Autodesk Inventor part; units mm, degrees
ref_plane "YZ Plane" through (0, 0, 0) normal (1, 0, 0) x (0, 1, 0)
ref_plane "XZ Plane" through (0, 0, 0) normal (0, 1, 0) x (-1, 0, 0)
ref_plane "XY Plane" through (0, 0, 0) normal (0, 0, 1) x (1, 0, 0)
sketch "Sketch1" plane through (0, 0, 0) normal (0, 0, 1) x (1, 0, 0)
  line L0 (0, 0) -> (300, 0)
  line L1 (300, 0) -> (300, 62)
  line L2 (300, 62) -> (0, 62)
  line L3 (0, 62) -> (0, 0)
  circle A0 centre (144.5, 55.5) radius 1.55
  circle A1 centre (144.5, 24.5) radius 1.55
  circle A2 centre (175.5, 55.5) radius 1.55
  circle A3 centre (175.5, 24.5) radius 1.55
  circle A4 centre (160, 40) radius 11.5
  line L4 (5, 19) -> (140, 19)
  line L5 (140, 19) -> (140, 15)
  line L6 (140, 15) -> (5, 15)
  line L7 (5, 15) -> (5, 19)
  line L8 (0, 62) -> (39.6145, 62)
  line L9 (8.1, 24.8) -> (5, 24.8)
  line L10 (5, 24.8) -> (5, 55.2)
  line L11 (5, 55.2) -> (8.1, 55.2)
  line L12 (8.1, 55.2) -> (8.1, 24.8)
  line L13 (8.1, 24.8) -> (5, 55.2) construction
  line L14 (5, 24.8) -> (8.1, 55.2) construction
  line L15 (0, 62) -> (50, 62)
  line L16 (0, 0) -> (0, -10)
  line L17 (0, -10) -> (300, -10)
  line L18 (300, -10) -> (300, 0)
  point P0 (6.55, 40)
  point P1 (5, 40)
  point P2 (8.1, 40)
  point P3 (5, 17)
  point P4 (140, 17)
  dimension "d1" = 3.1
  dimension "d2" = 3.1
  dimension "d3" = 3.1
  dimension "d4" = 3.1
  dimension "d5" = 31
  dimension "d7" = 23
  dimension "d8" = 15.5
  dimension "d9" = 15.5
  dimension "d10" = 62
  dimension "d11" = 31
  dimension "d13" = 40
  dimension "d54" = 300
  dimension "d55" = 3.1
  dimension "d56" = 5
  dimension "d57" = 15.2
  dimension "d59" = 135
  dimension "d93" = 15
  dimension "d106" = 20
  dimension "d107" = 5
  dimension "d201" = 4
  dimension "d202" = 10
extrude "Extrusion1" add sketch "Sketch1" along normal blind 3
sketch "Sketch4" plane through (0, 0, 3) normal (0, 0, 1) x (1, 0, 0)
  line L0 (300, 62) -> (0, 62)
  line L1 (244, 62) -> (248, 72)
  line L2 (248, 72) -> (254, 72)
  line L3 (254, 72) -> (250, 62)
  line L4 (0, -10) -> (300, -10)
  point P0 (0, 0)
  dimension "d108" = 10
  dimension "d109" = 4
  dimension "d110" = 50
  dimension "d111" = 6
extrude "Extrusion4" add sketch "Sketch4" against normal blind 3
sketch "Sketch7" plane through (0, 0, 3) normal (0, 0, 1) x (1, 0, 0)
  line L0 (134.4, 59.6) -> (137.6, 59.6)
  line L1 (137.6, 59.6) -> (137.6, 44.4)
  line L2 (137.6, 44.4) -> (134.4, 44.4)
  line L3 (134.4, 44.4) -> (134.4, 59.6)
  line L4 (134.4, 59.6) -> (137.6, 44.4) construction
  line L5 (137.6, 59.6) -> (134.4, 44.4) construction
  line L6 (134.4, 32.1) -> (137.6, 32.1)
  line L7 (137.6, 32.1) -> (137.6, 21.9)
  line L8 (137.6, 21.9) -> (134.4, 21.9)
  line L9 (134.4, 21.9) -> (134.4, 32.1)
  line L10 (134.4, 32.1) -> (137.6, 21.9) construction
  line L11 (137.6, 32.1) -> (134.4, 21.9) construction
  line L12 (244, 62) -> (0, 62)
  circle A0 centre (144.5, 55.5) radius 1.55
  line L13 (124.4, 59.6) -> (127.6, 59.6)
  line L14 (127.6, 59.6) -> (127.6, 44.4)
  line L15 (127.6, 44.4) -> (124.4, 44.4)
  line L16 (124.4, 44.4) -> (124.4, 59.6)
  line L17 (124.4, 59.6) -> (127.6, 44.4) construction
  line L18 (127.6, 59.6) -> (124.4, 44.4) construction
  line L19 (124.4, 32.1) -> (127.6, 32.1)
  line L20 (127.6, 32.1) -> (127.6, 21.9)
  line L21 (127.6, 21.9) -> (124.4, 21.9)
  line L22 (124.4, 21.9) -> (124.4, 32.1)
  line L23 (124.4, 32.1) -> (127.6, 21.9) construction
  line L24 (127.6, 32.1) -> (124.4, 21.9) construction
  line L25 (114.4, 59.6) -> (117.6, 59.6)
  line L26 (117.6, 59.6) -> (117.6, 44.4)
  line L27 (117.6, 44.4) -> (114.4, 44.4)
  line L28 (114.4, 44.4) -> (114.4, 59.6)
  line L29 (114.4, 59.6) -> (117.6, 44.4) construction
  line L30 (117.6, 59.6) -> (114.4, 44.4) construction
  line L31 (114.4, 32.1) -> (117.6, 32.1)
  line L32 (117.6, 32.1) -> (117.6, 21.9)
  line L33 (117.6, 21.9) -> (114.4, 21.9)
  line L34 (114.4, 21.9) -> (114.4, 32.1)
  line L35 (114.4, 32.1) -> (117.6, 21.9) construction
  line L36 (117.6, 32.1) -> (114.4, 21.9) construction
  line L37 (104.4, 59.6) -> (107.6, 59.6)
  line L38 (107.6, 59.6) -> (107.6, 44.4)
  line L39 (107.6, 44.4) -> (104.4, 44.4)
  line L40 (104.4, 44.4) -> (104.4, 59.6)
  line L41 (104.4, 59.6) -> (107.6, 44.4) construction
  line L42 (107.6, 59.6) -> (104.4, 44.4) construction
  line L43 (104.4, 32.1) -> (107.6, 32.1)
  line L44 (107.6, 32.1) -> (107.6, 21.9)
  line L45 (107.6, 21.9) -> (104.4, 21.9)
  line L46 (104.4, 21.9) -> (104.4, 32.1)
  line L47 (104.4, 32.1) -> (107.6, 21.9) construction
  line L48 (107.6, 32.1) -> (104.4, 21.9) construction
  line L49 (94.4, 59.6) -> (97.6, 59.6)
  line L50 (97.6, 59.6) -> (97.6, 44.4)
  line L51 (97.6, 44.4) -> (94.4, 44.4)
  line L52 (94.4, 44.4) -> (94.4, 59.6)
  line L53 (94.4, 59.6) -> (97.6, 44.4) construction
  line L54 (97.6, 59.6) -> (94.4, 44.4) construction
  line L55 (94.4, 32.1) -> (97.6, 32.1)
  line L56 (97.6, 32.1) -> (97.6, 21.9)
  line L57 (97.6, 21.9) -> (94.4, 21.9)
  line L58 (94.4, 21.9) -> (94.4, 32.1)
  line L59 (94.4, 32.1) -> (97.6, 21.9) construction
  line L60 (97.6, 32.1) -> (94.4, 21.9) construction
  line L61 (134.4, 10.1) -> (137.6, 10.1)
  line L62 (137.6, 10.1) -> (137.6, -0.1)
  line L63 (137.6, -0.1) -> (134.4, -0.1)
  line L64 (134.4, -0.1) -> (134.4, 10.1)
  line L65 (134.4, 10.1) -> (137.6, -0.1) construction
  line L66 (137.6, 10.1) -> (134.4, -0.1) construction
  line L67 (127.6, 10.1) -> (127.6, -0.1)
  line L68 (127.6, -0.1) -> (124.4, -0.1)
  line L69 (124.4, 10.1) -> (127.6, 10.1)
  line L70 (124.4, -0.1) -> (124.4, 10.1)
  line L71 (124.4, 10.1) -> (127.6, -0.1) construction
  line L72 (127.6, 10.1) -> (124.4, -0.1) construction
  line L73 (117.6, 10.1) -> (117.6, -0.1)
  line L74 (117.6, -0.1) -> (114.4, -0.1)
  line L75 (114.4, 10.1) -> (117.6, 10.1)
  line L76 (114.4, -0.1) -> (114.4, 10.1)
  line L77 (114.4, 10.1) -> (117.6, -0.1) construction
  line L78 (117.6, 10.1) -> (114.4, -0.1) construction
  line L79 (107.6, 10.1) -> (107.6, -0.1)
  line L80 (107.6, -0.1) -> (104.4, -0.1)
  line L81 (104.4, 10.1) -> (107.6, 10.1)
  line L82 (104.4, -0.1) -> (104.4, 10.1)
  line L83 (104.4, 10.1) -> (107.6, -0.1) construction
  line L84 (107.6, 10.1) -> (104.4, -0.1) construction
  line L85 (97.6, 10.1) -> (97.6, -0.1)
  line L86 (97.6, -0.1) -> (94.4, -0.1)
  line L87 (94.4, 10.1) -> (97.6, 10.1)
  line L88 (94.4, -0.1) -> (94.4, 10.1)
  line L89 (94.4, 10.1) -> (97.6, -0.1) construction
  line L90 (97.6, 10.1) -> (94.4, -0.1) construction
  line L91 (0, -10) -> (300, -10)
  line L92 (300, -10) -> (300, 62)
  point P0 (0, 0)
  point P1 (136, 52)
  point P2 (136, 27)
  point P3 (126, 52)
  point P4 (126, 27)
  point P5 (116, 52)
  point P6 (116, 27)
  point P7 (106, 52)
  point P8 (106, 27)
  point P9 (96, 52)
  point P10 (96, 27)
  point P11 (134.4, 52)
  point P12 (114.4, 52)
  point P13 (136, 5)
  point P14 (126, 5)
  point P15 (116, 5)
  point P16 (106, 5)
  point P17 (96, 5)
  point P18 (134.4, 5)
  point P19 (114.4, 5)
  point P20 (150, -10)
  dimension "d147" = 3.2
  dimension "d148" = 15.2
  dimension "d149" = 10.2
  dimension "d150" = 25
  dimension "d151" = 10
  dimension "d153" = 3.2
  dimension "d154" = 15.2
  dimension "d155" = 10.2
  dimension "d156" = 25
  dimension "d157" = 3.2
  dimension "d158" = 15.2
  dimension "d159" = 10.2
  dimension "d160" = 25
  dimension "d161" = 3.2
  dimension "d162" = 15.2
  dimension "d163" = 10.2
  dimension "d164" = 25
  dimension "d165" = 3.2
  dimension "d166" = 15.2
  dimension "d167" = 10.2
  dimension "d168" = 25
  dimension "d169" = 10
  dimension "d170" = 10
  dimension "d171" = 10
  dimension "d172" = 10
  dimension "d181" = 3.2
  dimension "d183" = 3.2
  dimension "d185" = 3.2
  dimension "d187" = 3.2
  dimension "d189" = 3.2
  dimension "d191" = 10
  dimension "d192" = 10
  dimension "d193" = 10
  dimension "d194" = 10
  dimension "d234" = 15
  dimension "d235" = 10.2
  dimension "d245" = 164
extrude "Extrusion6" cut sketch "Sketch7" against normal blind 3 contours L0 L1 L2 L3 | L6 L7 L8 L9 | L13 L14 L15 L16 | L19 L20 L21 L22 | L25 L26 L27 L28 | L31 L32 L33 L34 | L37 L38 L39 L40 | L43 L44 L45 L46 | L49 L50 L51 L52 | L55 L56 L57 L58 | L61 L62 L63 L64 | L67 L68 L70 L69 | L73 L74 L76 L75 | L79 L80 L82 L81 | L85 L86 L88 L87
sketch "Sketch8" plane through (0, 0, 3) normal (0, 0, 1) x (1, 0, 0)
  line L0 (0, -10) -> (300, -10)
  line L1 (279.8, 18) -> (290, 18)
  line L2 (290, 18) -> (290, 14.8)
  line L3 (290, 14.8) -> (279.8, 14.8)
  line L4 (279.8, 14.8) -> (279.8, 18)
  line L5 (300, -10) -> (300, 62)
  line L6 (4, 11.2) -> (7.2, 11.2)
  line L7 (7.2, 11.2) -> (7.2, -4)
  line L8 (7.2, -4) -> (4, -4)
  line L9 (4, -4) -> (4, 11.2)
  line L10 (4, 11.2) -> (7.2, -4) construction
  line L11 (7.2, 11.2) -> (4, -4) construction
  line L12 (282.4, 10.1) -> (285.6, 10.1)
  line L13 (285.6, 10.1) -> (285.6, -0.1)
  line L14 (285.6, -0.1) -> (282.4, -0.1)
  line L15 (282.4, -0.1) -> (282.4, 10.1)
  line L16 (282.4, 10.1) -> (285.6, -0.1) construction
  line L17 (285.6, 10.1) -> (282.4, -0.1) construction
  line L18 (274.4, 10.1) -> (277.6, 10.1)
  line L19 (277.6, 10.1) -> (277.6, -0.1)
  line L20 (277.6, -0.1) -> (274.4, -0.1)
  line L21 (274.4, -0.1) -> (274.4, 10.1)
  line L22 (274.4, 10.1) -> (277.6, -0.1) construction
  line L23 (277.6, 10.1) -> (274.4, -0.1) construction
  line L24 (97.6, -2.45) -> (282.4, -2.45)
  line L25 (282.4, -2.45) -> (282.4, -5.55)
  line L26 (282.4, -5.55) -> (97.6, -5.55)
  line L27 (97.6, -5.55) -> (97.6, -2.45)
  line L28 (97.6, -2.45) -> (282.4, -5.55) construction
  line L29 (282.4, -2.45) -> (97.6, -5.55) construction
  line L30 (137.6, 10.1) -> (137.6, -0.1)
  line L31 (290.4, 12.2) -> (293.6, 12.2)
  line L32 (293.6, 12.2) -> (293.6, -3)
  line L33 (293.6, -3) -> (290.4, -3)
  line L34 (290.4, -3) -> (290.4, 12.2)
  line L35 (290.4, 12.2) -> (293.6, -3) construction
  line L36 (293.6, 12.2) -> (290.4, -3) construction
  point P0 (0, 0)
  point P1 (5.6, 3.6)
  point P2 (4, 3.6)
  point P3 (284, 5)
  point P4 (282.4, 5)
  point P5 (276, 5)
  point P6 (274.4, 5)
  point P7 (190, -4)
  point P8 (137.6, 5)
  point P9 (97.6, -0.1)
  point P10 (292, 4.6)
  dimension "d219" = 28
  dimension "d220" = 3.2
  dimension "d221" = 10.2
  dimension "d222" = 10
  dimension "d223" = 3.2
  dimension "d224" = 15.2
  dimension "d225" = 4
  dimension "d226" = 6
  dimension "d227" = 3.2
  dimension "d229" = 3.2
  dimension "d232" = 8
  dimension "d233" = 15
  dimension "d236" = 3.1
  dimension "d237" = 9
  dimension "d238" = 10.2
  dimension "d240" = 3.2
  dimension "d241" = 15.2
  dimension "d242" = 7
  dimension "d243" = 16
  dimension "d244" = 8
extrude "Extrusion7" cut sketch "Sketch8" against normal blind 3
properties part number "Sideboard"
Check sheet for the modelled part. Datum: model origin and axes. Units: mm. Give positions to 0.01 mm unless a question says otherwise; leave off trailing zeros. Order: outer loops, then holes, each group sorted by start corner. A loop starts at its lowest first (then second) coordinate and runs counter-clockwise, first axis right, second up. Notation, with made-up numbers: M 28.5,12 L 59.5,12 A20 cw 59.5,47 Z; hole C -10,29 d7. An arc over 180 degrees is marked long. Answer as CSV lines item,"result". Start each with the question number.
Item 1: Gauge pin test, flat end, axial feed: P1, Ø1.5, axis at x = 136, z = 1.5, coming from the +Y side. Record the tip position at first contact, or that the pin passes through.
Item 2: Cross-section at C-C on x = 160. Enter the section's corners in (y, z).
Item 3: Cross-section at A-A on y = 40. Enter the section's corners in (x, z), plus the area to 3 significant figures.
Item 4: Mould release check, pull along Y, two halves, no side actions. Record for faces 1 (the face through (148, 32, 3)), 2 (the face through (148.51, 39.49, 1.48)): +Y half, -Y half, draft (parallel to the pull), parting line (faces both ways), or undercut.
Item 5: Cross-section at B-B on x = 197.5. Enter the section's corners in (y, z), plus the area to 3 significant figures.
Item 6: Thickness scan on line 1 (Y direction, x = 175.5, z = 0.8); line 2 (Y direction, x = 160, z = 0.6); line 3 (Y direction, x = 55.5, z = 2.2). Record the ranges inside material, lowest first. Write a range as [from, to].
Item 7: Cross-section at D-D on x = 53.5. Enter the section's corners in (y, z), plus the area to 3 significant figures.
Established:
1,P1,"stops at y = 62"
2,outline,"M -10,0 L -5.55,0 L -5.55,3 L -10,3 Z; M -2.45,0 L 28.5,0 L 28.5,3 L -2.45,3 Z; M 51.5,0 L 62,0 L 62,3 L 51.5,3 Z"
3,outline,"M 0,0 L 5,0 L 5,3 L 0,3 Z; M 8.1,0 L 148.5,0 L 148.5,3 L 8.1,3 Z; M 171.5,0 L 300,0 L 300,3 L 171.5,3 Z"
3,area,"822 mm^2"
4,face 1,"draft"
4,face 2,"undercut"
5,outline,"M -10,0 L -5.55,0 L -5.55,3 L -10,3 Z; M -2.45,0 L 62,0 L 62,3 L -2.45,3 Z"
5,area,"207 mm^2"
6,line 1,"y = [-10, -5.55], [-2.45, 22.95], [26.05, 53.95], [57.05, 62]"
6,line 2,"y = [-10, -5.55], [-2.45, 28.5], [51.5, 62]"
6,line 3,"y = [-10, 15], [19, 62]"
7,outline,"M -10,0 L 15,0 L 15,3 L -10,3 Z; M 19,0 L 62,0 L 62,3 L 19,3 Z"
7,area,"204 mm^2"
